CAD build for the part. Positions are in the model's coordinates, mm. A direction names the side the tool comes from. Coordinates: 2 decimals unless noted, no trailing zeros. Order: outer loops, then holes, each group sorted by start corner. A loop starts at its lowest first (then second) coordinate and runs counter-clockwise, first axis right, second up. Notation, with made-up numbers: M 26.25,54.5 L 43.25,54.5 A12 cw 43.25,61.5 Z; hole C -19.75,36.5 d11. An arc over 180 degrees is marked long. Write item = value, one per line.
from build123d import *

# Parameters (mm, degrees)
POCKET_DEPTH = 7.5
CHAMFER_SIZE = 1


with BuildPart() as part:
    # Sketch → Revolution (revolve)
    with BuildSketch(Plane.YZ):
        Polygon((2, 0), (9.7, 0), (9.25, 9), (7, 22.8), (2, 22.8), align=None)
    revolve(axis=Axis((0, 0, 0), (0, 0, 1)))

    # Sketch001 (on Face4 of Revolution) → Pocket (cut)
    with BuildSketch(Plane(origin=(0, 0, 22.8), x_dir=(0, -1, 0), z_dir=(0, 0, 1))):
        Polygon((4.041452, 0), (2.020726, 3.5), (-2.020726, 3.5), (-4.041452, 0), (-2.020726, -3.5), (2.020726, -3.5), align=None)
    extrude(amount=-POCKET_DEPTH, mode=Mode.SUBTRACT)

    # Chamfer
    chamfer_edges = [part.edges().sort_by_distance(p)[0] for p in [
        (0, -9.7, 0),
    ]]
    chamfer(chamfer_edges, length=CHAMFER_SIZE)


solid = part.part
(1) Slice it at C-C, the plane z = 6.75. Write the cut outline in (x, y) (1 decimal).
Evaluation:
outline = C 0,0 d18.7; hole C 0,0 d4
(2) Wall check: line 1 (Y direction, x = 0, z = 11.25); line 2 (Y direction, x = 0, z = 4.75); line 3 (X direction, y = 0, z = 4.5) (3 decimals). Give the ranges that are in metal, low to high. Write a range as from..to.
Evaluation:
line_1 = -8.88..-2, 2..8.88
line_2 = -9.46..-2, 2..9.46
line_3 = -9.475..-2, 2..9.475
(3) Slice it at B-B, the plane z = 21. Write the cut outline in (x, y).
Evaluation:
outline = C 0,0 d14.59; hole M -3.5,-2.02 L 0,-4.04 L 3.5,-2.02 L 3.5,2.02 L 0,4.04 L -3.5,2.02 Z
(4) Pin check, flat tips, straight feed: pin 1 Ø4.5 at (y, z) = (-0.5, 18) entering from +X; pin 2 Ø1 at (y, z) = (7, 4) entering from +X; pin 3 Ø2.5 at (x, y) = (0, 0) entering from +Z; pin 4 Ø3 at (y, z) = (-0.5, 18) entering from -X. Stop position of each tip, or through.
Evaluation:
pin_1 = 8.14
pin_2 = 6.93
pin_3 = through
pin_4 = -8.02
(5) Pull direction X, two halves, no side cores. Call faces 3 (the face through (9.18, -2.04, 5.94)), 4 (the face through (1.726, -3.045, 19.102)), 5 (the face through (-1.726, 3.045, 19.102)), 6 (the face through (2, -2, 0)): +X half, -X half, draft (parallel to the pull), parting line (faces both ways), or undercut.
Evaluation:
face_3 = parting line
face_4 = undercut
face_5 = undercut
face_6 = draft
(6) Slice it at A-A, the plane y = 0. Write the cut outline in (x, z).
Evaluation:
outline = M -9.65,1 L -8.7,0 L -2,0 L -2,15.3 L -3.5,15.3 L -3.5,22.8 L -7,22.8 L -9.25,9 Z; M 2,0 L 8.7,0 L 9.65,1 L 9.25,9 L 7,22.8 L 3.5,22.8 L 3.5,15.3 L 2,15.3 Z
(7) Tool access for faces 1 (the face through (2, 0, 8)), 2 (the face through (3.5, 0, 19)): list every direction of +Z, -Z, +X, -X, +Y, -Y with a clear straight run to the whole face (end or side of a thin tool).
Evaluation:
face_1 = +Z, -Z
face_2 = +Z
